Check sheet for the modelled part. Datum: model origin and axes. Units: mm. A direction names the side the tool comes from. Round coordinates to 2 decimals unless told otherwise and drop trailing zeros. Order: outer loops, then holes, each group sorted by start corner. A loop starts at its lowest first (then second) coordinate and runs counter-clockwise, first axis right, second up. Notation, with made-up numbers: (81.25, -22) -> (119.25, -22) arc R10 ccw to (119.25, -8) -> close; hole circle Ø11 at (76.5, -32.5). An arc over 180 degrees is marked (long way). Answer in a Markdown table with one row per item.
```python
from build123d import *

# Parameters (mm, degrees)
SKETCH5_W     = 1.5
SKETCH5_H     = 6.23
CHAMFER1_SIZE = 0.0635
CHAMFER2_SIZE = 0.1925


with BuildPart() as part:
    # Sketch3 → Revolve1 (revolve)
    with BuildSketch(Plane.XY, mode=Mode.PRIVATE) as revolve1_sk:
        Polygon((0, 0), (1.95, 0), (1.95, 0.53), (1.725, 0.53), (1.725, 0.71), (2.35, 0.71), (2.35, 3.07), (1.725, 3.07), (1.725, 3.25), (2.35, 3.25), (2.35, 5.61), (1.725, 5.61), (1.725, 5.7), (2.75, 5.7), (2.75, 6.23), (0, 6.23), align=None)
    revolve(revolve1_sk.sketch.rotate(Axis((0, 0, 0), (0, 1, 0)), 90), axis=Axis((0, 0, 0), (0, 1, 0)))

    # Sketch5 → Cut-Revolve1 (revolve, cut)
    with BuildSketch(Plane.XY, mode=Mode.PRIVATE) as cut_revolve1_sk:
        with Locations((0.75, 3.115)):
            Rectangle(SKETCH5_W, SKETCH5_H)
    revolve(cut_revolve1_sk.sketch.rotate(Axis((0, 0, 0), (0, 1, 0)), 90), axis=Axis((0, 0, 0), (0, 1, 0)), mode=Mode.SUBTRACT)

    # Chamfer1
    chamfer1_edges = [part.edges().sort_by_distance(p)[0] for p in [
        (0, 5.61, 2.35),
        (0, 3.07, 2.35),
    ]]
    chamfer(chamfer1_edges, length=CHAMFER1_SIZE)

    # Chamfer2
    chamfer2_edges = [part.edges().sort_by_distance(p)[0] for p in [
        (0, 6.23, 2.75),
        (0, 0.71, 2.35),
    ]]
    chamfer(chamfer2_edges, length=CHAMFER2_SIZE)


solid = part.part
```
(1) Depth check by flat-ended pin: pin 1 Ø2 at (x, y) = (2, 2.5) entering from -Z; pin 2 Ø1.5 at (y, z) = (5.5, 1.5) entering from -X. Enter the tip coordinate at first touch or a pass-through.
Solutions:
| item | result |
|---|---|
| pin 1 | z = -2.13 |
| pin 2 | x = -2.64 |
(2) Tool access check on faces 4 (the cylindrical face through (2.685, 5.871, 0.596)), 5 (the cylindrical face through (2.294, 4.414, 0.509)), 6 (the flat face through (-2, 3.07, 0)). Record the directions out of +Z, -Z, +X, -X, +Y, -Y that give a thin tool (end or side, any length) a straight path to the whole face; none if there is none.
Solutions:
| item | result |
|---|---|
| face 4 | +Y, -Y |
| face 5 | -Y |
| face 6 | none |
(3) Draft check along X on faces 1 (the flat face through (-2, 3.25, 0)), 2 (the cylindrical face through (2.294, 1.969, 0.509)), 3 (the cylindrical face through (-0.45, 3.16, -1.43)). Enter one of: pulls with the +X half, pulls with the -X half, needs draft (parallel to the pull), parting line crosses it, or undercut.
Solutions:
| item | result |
|---|---|
| face 1 | needs draft |
| face 2 | parting line crosses it |
| face 3 | undercut |
(4) Scan lines: probe 1 along X at (y, z) = (1.5, 0); probe 2 along Z at (x, y) = (1.1, 4); probe 3 along X at (y, z) = (4.25, 0.4). Record each from-to range of solid material in increasing order. Write a range as from..to.
Solutions:
| item | result |
|---|---|
| probe 1 | -2.35..-1.5, 1.5..2.35 |
| probe 2 | -2.08..-1.02, 1.02..2.08 |
| probe 3 | -2.32..-1.45, 1.45..2.32 |
(5) Section check A-A on y = 3.75. Record the boundary of the cut face in (x, z).
Solutions:
| item | result |
|---|---|
| outline | circle Ø4.7 at (0, 0); hole circle Ø3 at (0, 0) |
